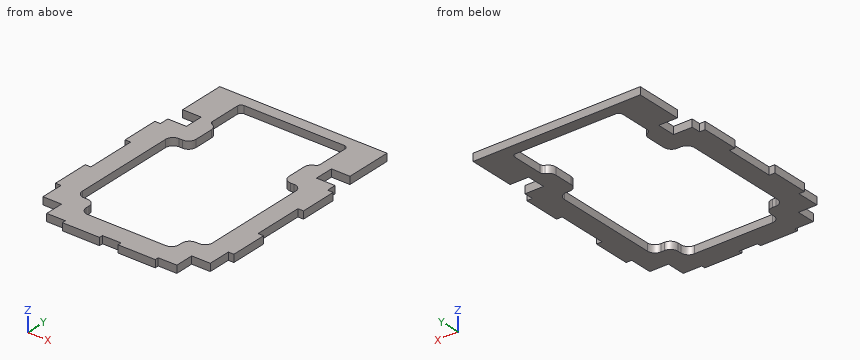
from build123d import *

# Parameters (mm, degrees)
EXTRUDE_1_DEPTH = 2


with BuildPart() as part:
    # Model → 凸台-拉伸1 (new body)
    with BuildSketch(Plane.XY):
        Polygon((1254.914320118, 540.768046392), (1254.914320118, 528.295619897), (1259.914320118, 528.295619897), (1259.914320118, 523.295619897), (1254.914320118, 523.295619897), (1254.914320118, 520.800244347), (1253.414320118, 520.800244347), (1253.414320118, 510.800244347), (1254.914320118, 510.800244347), (1254.914320118, 497.378469897), (1253.414320118, 497.378469897), (1253.414320118, 487.378469897), (1254.914320118, 487.378469897), (1254.914320118, 481.295619897), (1259.914320118, 481.295619897), (1259.914320118, 476.295619897), (1264.914320118, 476.295619897), (1264.914320118, 475.295619897), (1274.914320118, 475.295619897), (1274.914320118, 476.295619897), (1279.914320118, 476.295619897), (1279.914320118, 475.295619897), (1289.914320118, 475.295619897), (1289.914320118, 476.295619897), (1294.914320118, 476.295619897), (1294.914320118, 481.295619897), (1299.914320118, 481.295619897), (1299.914320118, 487.378469897), (1301.414320118, 487.378469897), (1301.414320118, 497.378469897), (1299.914320118, 497.378469897), (1299.914320118, 510.800244347), (1301.414320118, 510.800244347), (1301.414320118, 520.800244347), (1299.914320118, 520.800244347), (1299.914320118, 523.295619897), (1294.914320118, 523.295619897), (1294.914320118, 528.295619897), (1299.914320118, 528.295619897), (1299.914320118, 540.768046392), align=None)
        with BuildLine():
            Line((1264.914320118, 525.425619897), (1264.914320118, 520.295619897))
            ThreePointArc((1264.914320118, 520.295619897), (1264.32853368, 518.881406334), (1262.914320118, 518.295619897))
            Line((1262.914320118, 518.295619897), (1261.914320118, 518.295619897))
            ThreePointArc((1261.914320118, 518.295619897), (1260.500106556, 517.709833459), (1259.914320118, 516.295619897))
            Line((1259.914320118, 516.295619897), (1259.914320118, 488.295619897))
            ThreePointArc((1259.914320118, 488.295619897), (1260.500106556, 486.881406334), (1261.914320118, 486.295619897))
            Line((1261.914320118, 486.295619897), (1262.914320118, 486.295619897))
            ThreePointArc((1262.914320118, 486.295619897), (1264.32853368, 485.709833459), (1264.914320118, 484.295619897))
            Line((1264.914320118, 484.295619897), (1264.914320118, 483.295619897))
            ThreePointArc((1264.914320118, 483.295619897), (1265.500106556, 481.881406334), (1266.914320118, 481.295619897))
            Line((1266.914320118, 481.295619897), (1287.914320118, 481.295619897))
            ThreePointArc((1287.914320118, 481.295619897), (1289.32853368, 481.881406334), (1289.914320118, 483.295619897))
            Line((1289.914320118, 483.295619897), (1289.914320118, 484.295619897))
            ThreePointArc((1289.914320118, 484.295619897), (1290.500106556, 485.709833459), (1291.914320118, 486.295619897))
            Line((1291.914320118, 486.295619897), (1292.914320118, 486.295619897))
            ThreePointArc((1292.914320118, 486.295619897), (1294.32853368, 486.881406334), (1294.914320118, 488.295619897))
            Line((1294.914320118, 488.295619897), (1294.914320118, 516.295619897))
            ThreePointArc((1294.914320118, 516.295619897), (1294.32853368, 517.709833459), (1292.914320118, 518.295619897))
            Line((1292.914320118, 518.295619897), (1291.914320118, 518.295619897))
            ThreePointArc((1291.914320118, 518.295619897), (1290.500106556, 518.881406334), (1289.914320118, 520.295619897))
            Line((1289.914320118, 520.295619897), (1289.914320118, 525.425619897))
            ThreePointArc((1289.914320118, 525.425619897), (1290.281326956, 526.580320435), (1291.247653451, 527.31123798))
            ThreePointArc((1291.247653451, 527.31123798), (1291.730816699, 527.676696752), (1291.914320118, 528.254047021))
            Line((1291.914320118, 528.254047021), (1291.914320118, 536.716299759))
            ThreePointArc((1291.914320118, 536.716299759), (1291.621426899, 537.42340654), (1290.914320118, 537.716299759))
            Line((1290.914320118, 537.716299759), (1263.914320118, 537.716299759))
            ThreePointArc((1263.914320118, 537.716299759), (1263.207213337, 537.42340654), (1262.914320118, 536.716299759))
            Line((1262.914320118, 536.716299759), (1262.914320118, 528.254047021))
            ThreePointArc((1262.914320118, 528.254047021), (1263.097823537, 527.676696752), (1263.580986785, 527.31123798))
            ThreePointArc((1263.580986785, 527.31123798), (1264.54731328, 526.580320435), (1264.914320118, 525.425619897))
        make_face(mode=Mode.SUBTRACT)
    extrude(amount=EXTRUDE_1_DEPTH)


solid = part.part
Read the model definition and answer for the solid it produces. Units are mm, in the model's axes. Round coordinates to 2 decimals unless told otherwise and drop trailing zeros. Write each loop counter-clockwise with the first axis right and the second up, starting at its lowest first coordinate (ties: lowest second). Pieces come first, ordered by that corner, then holes. Notation, with made-up numbers: (-36.75, 19) - (-12.75, 19) arc R32 cw to (-12.75, 57) - close; hole circle Ø3 at (48, 34.25). An arc over 180 degrees is marked (long way). One line per question, with ' | ' between items. Start each with the question number.
1. Section B-B (x = 1273) is taken. Determine the outline of the cut face in (y, z).
2. Section A-A (y = 503) is taken. Determine the outline of the cut face in (x, z), and give its area (3 significant figures).
3. Each of these flat-tipped pins is pushed along its axis until it touches: pin 1 (0.6 mm diameter, centred on y = 522, z = 1.5, fed in from -X); pin 2 (1 mm diameter, centred on x = 1292, z = 0.5, fed in from -Y); pin 3 (0.6 mm diameter, centred on y = 525.5, z = 1, fed in from +X). Where does it stop, or does it pass through?
4. Find the intervals of material crossed by probe 1 along Y at (x, z) = (1270, 0.65); probe 2 along X at (y, z) = (520.5, 1.05); probe 3 along X at (y, z) = (499.5, 1.6), in increasing order. Write a range as [from, to].
Filled in:
1) outline: (475.3, 0) - (481.3, 0) - (481.3, 2) - (475.3, 2) - close; (537.72, 0) - (540.77, 0) - (540.77, 2) - (537.72, 2) - close
2) outline: (1254.91, 0) - (1259.91, 0) - (1259.91, 2) - (1254.91, 2) - close; (1294.91, 0) - (1299.91, 0) - (1299.91, 2) - (1294.91, 2) - close | area: 20.0 mm²
3) pin 1: x = 1254.91 | pin 2: y = 476.3 | pin 3: x = 1294.91
4) probe 1: [475.3, 481.3], [537.72, 540.77] | probe 2: [1253.41, 1264.91], [1289.91, 1301.41] | probe 3: [1254.91, 1259.91], [1294.91, 1299.91]
